Geometry check sheet. Reference: the model listing, model coordinates, mm. Face numbers are marked on the shaded views. Round coordinates to 2 decimals unless told otherwise and drop trailing zeros. Loops run counter-clockwise (first coordinate to the right, second up) from the corner with the lowest first, then second, coordinate; pieces in that order, holes last. Notation, with made-up numbers: (-1, -15.75) -> (46, -15.75) arc R18 cw to (46, 3.25) -> close; hole circle Ø1 at (2, 61.5). An arc over 180 degrees is marked (long way). Use one line per item in the form item = value.
from build123d import *

# Parameters (mm, degrees)
SKETCH1_R           = 60
SKETCH1_R_2         = 26.1
SKETCH1_R_3         = 2.6
BOSS_EXTRUDE1_DEPTH = 8
SKETCH2_R           = 60
SKETCH2_R_2         = 40
SKETCH2_R_3         = 2.6
BOSS_EXTRUDE2_DEPTH = 8
SKETCH3_R           = 4.6
SKETCH3_R_2         = 2.6
BOSS_EXTRUDE3_DEPTH = 4.8
SKETCH4_R           = 26.1
SKETCH4_R_2         = 22.5
BOSS_EXTRUDE4_DEPTH = 1
CHAMFER1_SIZE       = 1
SKETCH5_R           = 4.6
SKETCH5_R_2         = 2.6
CUT_EXTRUDE1_DEPTH  = 7


with BuildPart() as part:
    # Sketch1 → Boss-Extrude1 (new body)
    with BuildSketch(Plane(origin=(0, 0, 0), x_dir=(1, 0, 0), z_dir=(0, 1, 0))):
        Circle(SKETCH1_R)
        Circle(SKETCH1_R_2, mode=Mode.SUBTRACT)
        with Locations((0, 50)):
            Circle(SKETCH1_R_3, mode=Mode.SUBTRACT)
        with Locations((23.236158602, 44.272801283)):
            Circle(SKETCH1_R_3, mode=Mode.SUBTRACT)
        with Locations((41.149193295, 28.403237337)):
            Circle(SKETCH1_R_3, mode=Mode.SUBTRACT)
        with Locations((49.635443705, 6.026834013)):
            Circle(SKETCH1_R_3, mode=Mode.SUBTRACT)
        with Locations((46.750812134, -17.730244352)):
            Circle(SKETCH1_R_3, mode=Mode.SUBTRACT)
        with Locations((33.156132912, -37.425537409)):
            Circle(SKETCH1_R_3, mode=Mode.SUBTRACT)
        with Locations((11.965783214, -48.547090871)):
            Circle(SKETCH1_R_3, mode=Mode.SUBTRACT)
        with Locations((-11.965783214, -48.547090871)):
            Circle(SKETCH1_R_3, mode=Mode.SUBTRACT)
        with Locations((-33.156132912, -37.425537409)):
            Circle(SKETCH1_R_3, mode=Mode.SUBTRACT)
        with Locations((-46.750812134, -17.730244352)):
            Circle(SKETCH1_R_3, mode=Mode.SUBTRACT)
        with Locations((-49.635443705, 6.026834013)):
            Circle(SKETCH1_R_3, mode=Mode.SUBTRACT)
        with Locations((-41.149193295, 28.403237337)):
            Circle(SKETCH1_R_3, mode=Mode.SUBTRACT)
        with Locations((-23.236158602, 44.272801283)):
            Circle(SKETCH1_R_3, mode=Mode.SUBTRACT)
    extrude(amount=BOSS_EXTRUDE1_DEPTH)

    # Sketch2 → Boss-Extrude2 (add)
    with BuildSketch(Plane(origin=(0, 0, 0), x_dir=(-1, 0, 0), z_dir=(0, -1, 0))):
        Circle(SKETCH2_R)
        Circle(SKETCH2_R_2, mode=Mode.SUBTRACT)
        with Locations((23.236158602, 44.272801283)):
            Circle(SKETCH2_R_3, mode=Mode.SUBTRACT)
        with Locations((41.149193295, 28.403237337)):
            Circle(SKETCH2_R_3, mode=Mode.SUBTRACT)
        with Locations((49.635443705, 6.026834013)):
            Circle(SKETCH2_R_3, mode=Mode.SUBTRACT)
        with Locations((46.750812134, -17.730244352)):
            Circle(SKETCH2_R_3, mode=Mode.SUBTRACT)
        with Locations((33.156132912, -37.425537409)):
            Circle(SKETCH2_R_3, mode=Mode.SUBTRACT)
        with Locations((11.965783214, -48.547090871)):
            Circle(SKETCH2_R_3, mode=Mode.SUBTRACT)
        with Locations((-11.965783214, -48.547090871)):
            Circle(SKETCH2_R_3, mode=Mode.SUBTRACT)
        with Locations((-33.156132912, -37.425537409)):
            Circle(SKETCH2_R_3, mode=Mode.SUBTRACT)
        with Locations((-46.750812134, -17.730244352)):
            Circle(SKETCH2_R_3, mode=Mode.SUBTRACT)
        with Locations((-49.635443705, 6.026834013)):
            Circle(SKETCH2_R_3, mode=Mode.SUBTRACT)
        with Locations((-41.149193295, 28.403237337)):
            Circle(SKETCH2_R_3, mode=Mode.SUBTRACT)
        with Locations((-23.236158602, 44.272801283)):
            Circle(SKETCH2_R_3, mode=Mode.SUBTRACT)
        with Locations((0, 50)):
            Circle(SKETCH2_R_3, mode=Mode.SUBTRACT)
    extrude(amount=BOSS_EXTRUDE2_DEPTH)

    # Sketch3 → Boss-Extrude3 (add)
    with BuildSketch(Plane.XZ.offset(8)):
        with Locations((0, -50)):
            Circle(SKETCH3_R)
        with Locations((0, -50)):
            Circle(SKETCH3_R_2, mode=Mode.SUBTRACT)
        with Locations((41.149193295, -28.403237337)):
            Circle(SKETCH3_R)
        with Locations((41.149193295, -28.403237337)):
            Circle(SKETCH3_R_2, mode=Mode.SUBTRACT)
        with Locations((46.750812134, 17.730244352)):
            Circle(SKETCH3_R)
        with Locations((46.750812134, 17.730244352)):
            Circle(SKETCH3_R_2, mode=Mode.SUBTRACT)
        with Locations((11.965783214, 48.547090871)):
            Circle(SKETCH3_R)
        with Locations((11.965783214, 48.547090871)):
            Circle(SKETCH3_R_2, mode=Mode.SUBTRACT)
        with Locations((-33.156132912, 37.425537409)):
            Circle(SKETCH3_R)
        with Locations((-33.156132912, 37.425537409)):
            Circle(SKETCH3_R_2, mode=Mode.SUBTRACT)
        with Locations((-49.635443705, -6.026834013)):
            Circle(SKETCH3_R)
        with Locations((-49.635443705, -6.026834013)):
            Circle(SKETCH3_R_2, mode=Mode.SUBTRACT)
        with Locations((-23.236158602, -44.272801283)):
            Circle(SKETCH3_R)
        with Locations((-23.236158602, -44.272801283)):
            Circle(SKETCH3_R_2, mode=Mode.SUBTRACT)
        with Locations((-41.149193295, -28.403237337)):
            Circle(SKETCH3_R)
        with Locations((-41.149193295, -28.403237337)):
            Circle(SKETCH3_R_2, mode=Mode.SUBTRACT)
        with Locations((-46.750812134, 17.730244352)):
            Circle(SKETCH3_R)
        with Locations((-46.750812134, 17.730244352)):
            Circle(SKETCH3_R_2, mode=Mode.SUBTRACT)
        with Locations((-11.965783214, 48.547090871)):
            Circle(SKETCH3_R)
        with Locations((-11.965783214, 48.547090871)):
            Circle(SKETCH3_R_2, mode=Mode.SUBTRACT)
        with Locations((33.156132912, 37.425537409)):
            Circle(SKETCH3_R)
        with Locations((33.156132912, 37.425537409)):
            Circle(SKETCH3_R_2, mode=Mode.SUBTRACT)
        with Locations((49.635443705, -6.026834013)):
            Circle(SKETCH3_R)
        with Locations((49.635443705, -6.026834013)):
            Circle(SKETCH3_R_2, mode=Mode.SUBTRACT)
        with Locations((23.236158602, -44.272801283)):
            Circle(SKETCH3_R)
        with Locations((23.236158602, -44.272801283)):
            Circle(SKETCH3_R_2, mode=Mode.SUBTRACT)
    extrude(amount=BOSS_EXTRUDE3_DEPTH)

    # Sketch4 → Boss-Extrude4 (add)
    with BuildSketch(Plane(origin=(0, 8, 0), x_dir=(1, 0, 0), z_dir=(0, 1, 0))):
        Circle(SKETCH4_R)
        Circle(SKETCH4_R_2, mode=Mode.SUBTRACT)
    extrude(amount=-BOSS_EXTRUDE4_DEPTH)

    # Chamfer1
    chamfer1_edges = [part.edges().sort_by_distance(p)[0] for p in [
        (-26.1, 0, 0),
    ]]
    chamfer(chamfer1_edges, length=CHAMFER1_SIZE)

    # Sketch5 → Cut-Extrude1 (cut)
    with BuildSketch(Plane(origin=(0, 8, 0), x_dir=(1, 0, 0), z_dir=(0, 1, 0))):
        with Locations((-23.236158602, 44.272801283)):
            Circle(SKETCH5_R)
        with Locations((-23.236158602, 44.272801283)):
            Circle(SKETCH5_R_2, mode=Mode.SUBTRACT)
        with Locations((-49.635443705, 6.026834013)):
            Circle(SKETCH5_R)
        with Locations((-49.635443705, 6.026834013)):
            Circle(SKETCH5_R_2, mode=Mode.SUBTRACT)
        with Locations((-33.156132912, -37.425537409)):
            Circle(SKETCH5_R)
        with Locations((-33.156132912, -37.425537409)):
            Circle(SKETCH5_R_2, mode=Mode.SUBTRACT)
        with Locations((11.965783214, -48.547090871)):
            Circle(SKETCH5_R)
        with Locations((11.965783214, -48.547090871)):
            Circle(SKETCH5_R_2, mode=Mode.SUBTRACT)
        with Locations((46.750812134, -17.730244352)):
            Circle(SKETCH5_R)
        with Locations((46.750812134, -17.730244352)):
            Circle(SKETCH5_R_2, mode=Mode.SUBTRACT)
        with Locations((41.149193295, 28.403237337)):
            Circle(SKETCH5_R)
        with Locations((41.149193295, 28.403237337)):
            Circle(SKETCH5_R_2, mode=Mode.SUBTRACT)
        with Locations((0, 50)):
            Circle(SKETCH5_R)
        with Locations((0, 50)):
            Circle(SKETCH5_R_2, mode=Mode.SUBTRACT)
        with Locations((23.236158602, 44.272801283)):
            Circle(SKETCH5_R)
        with Locations((23.236158602, 44.272801283)):
            Circle(SKETCH5_R_2, mode=Mode.SUBTRACT)
        with Locations((49.635443705, 6.026834013)):
            Circle(SKETCH5_R)
        with Locations((49.635443705, 6.026834013)):
            Circle(SKETCH5_R_2, mode=Mode.SUBTRACT)
        with Locations((33.156132912, -37.425537409)):
            Circle(SKETCH5_R)
        with Locations((33.156132912, -37.425537409)):
            Circle(SKETCH5_R_2, mode=Mode.SUBTRACT)
        with Locations((-11.965783214, -48.547090871)):
            Circle(SKETCH5_R)
        with Locations((-11.965783214, -48.547090871)):
            Circle(SKETCH5_R_2, mode=Mode.SUBTRACT)
        with Locations((-46.750812134, -17.730244352)):
            Circle(SKETCH5_R)
        with Locations((-46.750812134, -17.730244352)):
            Circle(SKETCH5_R_2, mode=Mode.SUBTRACT)
        with Locations((-41.149193295, 28.403237337)):
            Circle(SKETCH5_R)
        with Locations((-41.149193295, 28.403237337)):
            Circle(SKETCH5_R_2, mode=Mode.SUBTRACT)
    extrude(amount=-CUT_EXTRUDE1_DEPTH, mode=Mode.SUBTRACT)


solid = part.part
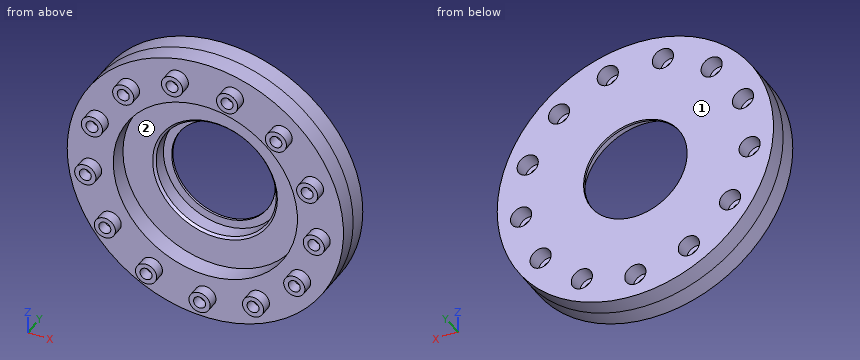
1. Gauge pin test, flat ends, axial feed: pin 1 (3 mm diameter, centred on y = -6, z = -6.5, fed in from +X); pin 2 (6 mm diameter, centred on x = -11.97, z = 48.55, fed in from +Y); pin 3 (10 mm diameter, centred on x = -11, y = -9, fed in from -Z). Record the tip position at first contact, or that the pin passes through.
Return value:
pin_1 = 59.79
pin_2 = 1
pin_3 = -59.69
2. Mould release check, pull along X, two halves, no side actions. Record for the marked faces 1 and 2: released by +X, released by -X, zero draft, split by the parting line, or undercut.
Return value:
face_1 = zero draft
face_2 = undercut
3. Section check C-C (z = 0). Record the boundary of the cut face in (x, y), then the cut area to 3 significant figures.
Return value:
outline = (-60, -8) -> (-40, -8) -> (-40, 0) -> (-27.1, 0) -> (-26.1, 1) -> (-26.1, 7) -> (-22.5, 7) -> (-22.5, 8) -> (-60, 8) -> close; (22.5, 7) -> (26.1, 7) -> (26.1, 1) -> (27.1, 0) -> (40, 0) -> (40, -8) -> (60, -8) -> (60, 8) -> (22.5, 8) -> close
area = 869 mm2
4. Material ranges on line 1 along Z through (x, y) = (0, 2.75); line 2 along Z through (x, y) = (49, 7); line 3 along X through (y, z) = (-9.5, -48.5), recorded low to high.
Return value:
line_1 = -60 to -54.6, -45.4 to -26.1, 26.1 to 60
line_2 = -34.63 to -10.58, -1.47 to 13.72, 21.74 to 34.63
line_3 = -25.05 to -21.42, -4.35 to -2.12, 2.12 to 4.35, 21.42 to 25.05
5. Section check A-A (x = 0). Count the separate pieces of the cut face and the enclosed holes in it, then the cut area to 3 significant figures.
Return value:
separate_pieces = 3
enclosed_holes = 0
area = 777 mm2
